CAD build for the part. Positions are in the model's coordinates, mm. A direction names the side the tool comes from. Give positions to 0.01 mm unless a question says otherwise; leave off trailing zeros. Loops run counter-clockwise (first coordinate to the right, second up) from the corner with the lowest first, then second, coordinate; pieces in that order, holes last. Notation, with made-up numbers: (1.25, 63) -> (19.25, 63) arc R17 cw to (19.25, 75) -> close; hole circle Ø4 at (24.5, 58). An arc over 180 degrees is marked (long way). Write each question's results on one line, items separated by ' | '. Start each with the question number.
Autodesk Inventor part; units mm, degrees
ref_plane "YZ Plane" through (0, 0, 0) normal (1, 0, 0) x (0, 1, 0)
ref_plane "XZ Plane" through (0, 0, 0) normal (0, 1, 0) x (-1, 0, 0)
sketch "Sketch2" plane through (0, 0, 0) normal (0, 0, 1) x (1, 0, 0)
  line L0 (5.0984, -40.3499) -> (19.0293, -40.3499)
  line L1 (22.6152, -35.9079) -> (22.6152, -8.9424)
  line L2 (18.9317, -4.3499) -> (5.0984, -4.3499)
  line L3 (1.5125, -8.792) -> (1.5125, -35.9079)
  line L4 (3.421, -5.2607) -> (1.8351, -7.7028)
  line L5 (3.421, -39.4392) -> (1.8351, -36.9971)
  line L6 (20.7066, -39.4392) -> (22.2925, -36.9971)
  line L7 (22.2925, -7.8531) -> (20.609, -5.2607)
  arc A0 (5.0984, -4.3499) -> (3.421, -5.2607) centre (5.0984, -6.3499) ccw
  arc A1 (1.8351, -7.7028) -> (1.5125, -8.792) centre (3.5125, -8.792) ccw
  arc A2 (20.609, -5.2607) -> (18.9317, -4.3499) centre (18.9317, -6.3499) ccw
  arc A3 (22.6152, -8.9424) -> (22.2925, -7.8531) centre (20.6152, -8.9424) ccw
  arc A4 (1.5125, -35.9079) -> (1.8351, -36.9971) centre (3.5125, -35.9079) ccw
  arc A5 (3.421, -39.4392) -> (5.0984, -40.3499) centre (5.0984, -38.3499) ccw
  arc A6 (19.0293, -40.3499) -> (20.7066, -39.4392) centre (19.0293, -38.3499) ccw
  arc A7 (22.2925, -36.9971) -> (22.6152, -35.9079) centre (20.6152, -35.9079) ccw
  point P0 (0, 0)
  point P1 (22.6152, -4.3499)
  point P2 (22.6152, -40.3499)
  dimension "d116" = 36
  dimension "d117" = 2
  dimension "d119" = 2
extrude "Extrusion1" add sketch "Sketch2" along normal blind 24
sketch "Sketch3" plane through (0, 0, 0) normal (0, 0, 1) x (1, 0, 0)
  circle A0 centre (12.015, -12.869) radius 8.5
  point P0 (0, 0)
  dimension "d244" = 17
extrude "Extrusion2" add sketch "Sketch3" against normal blind 3
sketch "Sketch6" plane through (0, 0, 0) normal (1, 0, 0) x (0, 1, 0)
  line L0 (-40.3499, 0) -> (-40.3499, 24)
  line L1 (-40.3499, 3) -> (-35.3499, 3)
  line L2 (-35.3499, 3) -> (-35.3499, 21)
  line L3 (-35.3499, 21) -> (-40.3499, 21)
  line L4 (-40.3499, 21) -> (-40.3499, 3)
  point P0 (0, 0)
  dimension "d221" = 5
  dimension "d222" = 18
extrude "Extrusion3" cut sketch "Sketch6" along normal up to next
ref_plane "Work Plane2" through (1.5125, -8.792, 24) normal (-1, 0, 0) x (0, -1, 0)
sketch "Sketch8" plane through (1.5125, -8.792, 24) normal (-1, 0, 0) x (0, -1, 0)
  line L0 (26.5579, -3) -> (26.5579, -21)
  line L1 (26.5579, -3) -> (1.5579, -3)
  line L2 (1.5579, -3) -> (1.5579, -21)
  line L3 (1.5579, -21) -> (26.5579, -21)
  line L4 (26.5579, -21) -> (26.5579, -3)
  dimension "d243" = 25
extrude "Extrusion4" add sketch "Sketch8" along normal blind 1.4485
ref_plane "Work Plane3" through (22.6152, -35.9079, 24) normal (1, 0, 0) x (0, 1, 0)
sketch "Sketch9" plane through (22.6152, -35.9079, 24) normal (1, 0, 0) x (0, 1, 0)
  line L0 (0.5579, -21) -> (25.5579, -21)
  line L1 (25.5579, -21) -> (25.5579, -3)
  line L2 (25.5579, -3) -> (0.5579, -3)
  line L3 (0.5579, -3) -> (0.5579, -21)
  dimension "d239" = 25
  dimension "d240" = 18
extrude "Extrusion5" add sketch "Sketch9" along normal blind 1.4485
sketch "Sketch10" plane through (0, 0, 0) normal (0, 0, 1) x (1, 0, 0)
  circle A0 centre (12.0638, -37.347) radius 2
  circle A1 centre (5.564, -37.347) radius 2
  circle A2 centre (18.564, -37.347) radius 2
  point P0 (0, 0)
  dimension "d245" = 4
  dimension "d246" = 4
  dimension "d247" = 4
extrude "Extrusion7" cut sketch "Sketch10" along normal blind 24
properties part number "servo"
Q1. Drop flat-ended pins along their axis: pin 1 (1.2 mm diameter, centred on x = 23.5, y = -20.5, fed in from -Z); pin 2 (12 mm diameter, centred on x = 11.5, y = -27.5, fed in from -Z); pin 3 (1.2 mm diameter, centred on x = 21, z = 16, fed in from -Y). Give the stop position or say it passes through.
Q2. Saw through at D-D, the plane x = 19.5. List the corners of the cut face in (y, z), then the cut area to 3 significant figures.
Q3. Saw through at A-A, the plane x = 10.75. List the corners of the cut face in (y, z).
Q4. Which spindle directions (+Z, -Z, +X, -X, +Y, -Y) get a long thin tool onto all of the face, cutting with end or side? Do faces 1 (the face through (23, -23, 3)), 2 (the face through (21, -35.35, 12)), 3 (the face through (1, -23, 3)), 4 (the face through (20.122, -10.316, -1.479)). Say none if no direction does.
Q5. Wall check: L1, parallel to Z at x = 20, y = -18.5; L2, parallel to Y at x = 18.5, z = 11.5; L3, parallel to X at y = -25, z = 22. Give the ranges that are in metal, low to high.
Q6. Saw through at C-C, the plane y = -25.5. List the corners of the cut face in (x, z).
Answer block:
1) pin 1: stops at z = 3 | pin 2: stops at z = 0 | pin 3: stops at y = -35.35
2) outline: (-40.29, 0) -> (-39.11, 0) -> (-39.11, 3) -> (-40.29, 3) -> close; (-40.29, 21) -> (-39.11, 21) -> (-39.11, 24) -> (-40.29, 24) -> close; (-35.58, 0) -> (-16.9, 0) -> (-16.9, -3) -> (-8.84, -3) -> (-8.84, 0) -> (-4.43, 0) -> (-4.43, 24) -> (-35.58, 24) -> (-35.58, 21) -> (-35.35, 21) -> (-35.35, 3) -> (-35.58, 3) -> close | area: 775 mm2
3) outline: (-40.35, 0) -> (-38.85, 0) -> (-38.85, 3) -> (-40.35, 3) -> close; (-40.35, 21) -> (-38.85, 21) -> (-38.85, 24) -> (-40.35, 24) -> close; (-35.84, 0) -> (-21.27, 0) -> (-21.27, -3) -> (-4.46, -3) -> (-4.46, 0) -> (-4.35, 0) -> (-4.35, 24) -> (-35.84, 24) -> (-35.84, 21) -> (-35.35, 21) -> (-35.35, 3) -> (-35.84, 3) -> close
4) face 1: -Z, +X, +Y, -Y | face 2: +X, -X, -Y | face 3: -Z, -X, +Y, -Y | face 4: -Z
5) L1: z = 0 to 24 | L2: y = -35.35 to -4.35 | L3: x = 1.51 to 22.62
6) outline: (0.06, 3) -> (1.51, 3) -> (1.51, 0) -> (22.62, 0) -> (22.62, 3) -> (24.06, 3) -> (24.06, 21) -> (22.62, 21) -> (22.62, 24) -> (1.51, 24) -> (1.51, 21) -> (0.06, 21) -> close
